Build history of the part. All positions in model axes, mm. Coordinates: 2 decimals unless noted, no trailing zeros. Loops run counter-clockwise (first coordinate to the right, second up) from the corner with the lowest first, then second, coordinate; pieces in that order, holes last.
(1) Wall check: L1, parallel to Y at x = 17, z = 2.3; L2, parallel to X at y = 7, z = 1.25; L3, parallel to X at y = 3, z = 1.45. Give the ranges that are in metal, low to high.
(2) Slice it at D-D (z = 0.85). Give the cut face in (x, y).
(3) Slice it at C-C (y = 39). Give the cut face in (x, z), and give its area (3 significant figures).
(4) Slice it at A-A (x = 17). Give the cut face in (y, z).
(5) Flat gauge pins, fed straight in: P1, Ø0.9, axis at y = 34.5, z = 1, coming from the +X side; P2, Ø1.5, axis at y = 7, z = 1.5, coming from the +X side; P3, Ø12, axis at x = 66, y = 20, coming from the +Z side. Where does each tip first touch, or does it go through?
(6) Slice it at B-B (y = 20). Give the cut face in (x, z), and give its area (4 significant figures).
Autodesk Inventor part; units mm, degrees
ref_plane "YZ Plane" through (0, 0, 0) normal (1, 0, 0) x (0, 1, 0)
ref_plane "XZ Plane" through (0, 0, 0) normal (0, 1, 0) x (-1, 0, 0)
ref_plane "XY Plane" through (0, 0, 0) normal (0, 0, 1) x (1, 0, 0)
sketch "Sketch1" plane through (0, 0, 0) normal (0, 0, 1) x (1, 0, 0)
  line L0 (0, 0) -> (40, 0)
  line L1 (40, 0) -> (40, 40)
  line L2 (40, 40) -> (0, 40)
  line L3 (0, 40) -> (0, 0)
  line L4 (40, 0) -> (37, 0)
  line L5 (37, 0) -> (37, 10)
  line L6 (37, 10) -> (40, 10)
  line L7 (40, 10) -> (40, 0)
  line L8 (40, 40) -> (37, 40)
  line L9 (37, 40) -> (37, 30)
  line L10 (37, 30) -> (40, 30)
  line L11 (40, 30) -> (40, 40)
  line L12 (0, -4) -> (40, -4)
  line L13 (40, -4) -> (40, 44)
  line L14 (40, 44) -> (0, 44)
  line L15 (0, 44) -> (0, -4)
  circle A0 centre (66, 20) radius 7.5
  circle A1 centre (66, 20) radius 12
  line L16 (40, -4) -> (70.6666, 8.9445)
  line L17 (40, 20) -> (43.7791, 20)
  line L18 (40, 44) -> (70.6666, 31.0555)
  circle A2 centre (17, 20) radius 4.25
  line L19 (37, 30) -> (37, 10)
  point P0 (20, 40)
  dimension "d0" = 40
  dimension "d1" = 40
  dimension "d2" = 3
  dimension "d3" = 10
  dimension "d4" = 10
  dimension "d5" = 4
  dimension "d6" = 4
  dimension "d7" = 15
  dimension "d8" = 24
  dimension "d9" = 26
  dimension "d11" = 8.5
  dimension "d17" = 20
  dimension "d18" = 20
extrude "Plate1" add sketch "Sketch1" along normal blind 3 contours L3 L2 L9 L19 L5 L0 | L0 L13 L12 L15 | L15 L14 L13 L2 | L1 L13 L18 A1 L16 | L19 L10 L1 L6 | A1
chamfer "Corner Chamfer1" distance 6 angle 45 2 edges at (0, 44, 1.5) (0, -4, 1.5)
equation "\"d6\" = d5"
equation "\"d10\" = Thickness"
equation "\"BendRadius\" = Thickness"
equation "\"BendReliefWidth\" = Thickness"
equation "\"BendReliefDepth\" = 0.5 * Thickness"
equation "\"CornerReliefSize\" = 4 * Thickness"
equation "\"MinimumRemnant\" = 2 * Thickness"
equation "\"TransitionRadius\" = BendRadius"
equation "\"JacobiRadiusSize\" = BendRadius"
equation "\"GapSize\" = Thickness"
properties part number "A_beam_piston_mount_2" material "Stainless Steel"
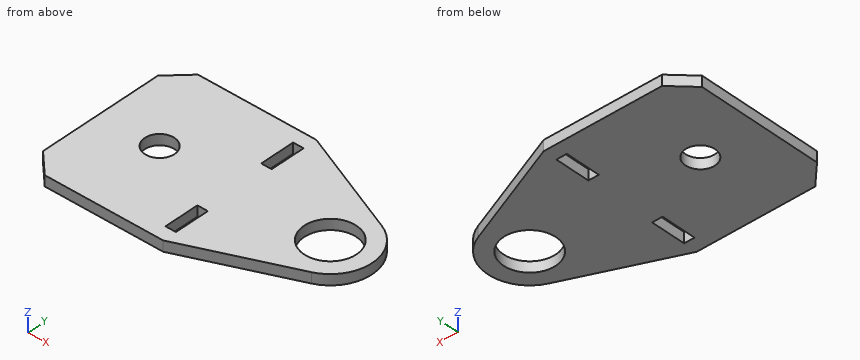
Response values:
1. L1: y = -4 to 15.75, 24.25 to 44
1. L2: x = 0 to 37, 40 to 66.06
1. L3: x = 0 to 37, 40 to 56.58
2. outline: (0, 2) - (6, -4) - (40, -4) - (70.67, 8.94) arc R12 ccw to (70.67, 31.06) - (40, 44) - (6, 44) - (0, 38) - close; hole circle Ø8.5 at (17, 20); hole (37, 0) - (40, 0) - (40, 10) - (37, 10) - close; hole (37, 30) - (40, 30) - (40, 40) - (37, 40) - close; hole circle Ø15 at (66, 20)
3. outline: (1, 0) - (37, 0) - (37, 3) - (1, 3) - close; (40, 0) - (51.85, 0) - (51.85, 3) - (40, 3) - close
3. area: 144 mm2
4. outline: (-4, 0) - (15.75, 0) - (15.75, 3) - (-4, 3) - close; (24.25, 0) - (44, 0) - (44, 3) - (24.25, 3) - close
5. P1: stops at x = 63.57
5. P2: stops at x = 67.84
5. P3: passes through
6. outline: (0, 0) - (12.75, 0) - (12.75, 3) - (0, 3) - close; (21.25, 0) - (58.5, 0) - (58.5, 3) - (21.25, 3) - close; (73.5, 0) - (78, 0) - (78, 3) - (73.5, 3) - close
6. area: 163.5 mm2
